Verification items for the finished model (mm, model axes). Face numbers are marked on the shaded views. A direction names the side the tool comes from. Give positions to 0.01 mm unless a question says otherwise; leave off trailing zeros. Write each loop counter-clockwise with the first axis right and the second up, starting at its lowest first coordinate (ties: lowest second). Pieces come first, ordered by that corner, then holes.
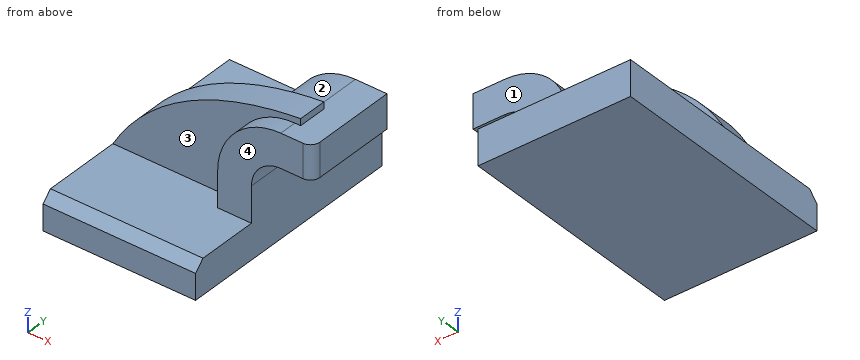
from build123d import *

# Parameters (mm, degrees)
F1_DEPTH = 63.5
F0_W     = 13.9366841115
F0_H     = 18.2897937342
F2_DEPTH = 25.4
F3_DEPTH = 15.875
F4_SIZE  = 5.08
F5_R     = 5.08


with BuildPart() as f1:
    # F0 (on Front) → F1 (new body, symmetric)
    with BuildSketch(Plane.XZ):
        Polygon((22.9852062658, 9.525), (-41.275, 9.525), (-41.275, -9.525), (41.275, -9.525), (41.275, 9.525), align=None)
    extrude(amount=F1_DEPTH, both=True)

    # F0 (on Front) → F2 (join, symmetric)
    with BuildSketch(Plane.XZ):
        with BuildLine():
            Line((22.9852062658, 28.8565382361), (22.9852062658, 9.525))
            Line((22.9852062658, 9.525), (41.275, 9.525))
            Line((41.275, 9.525), (41.275, 28.8565382361))
            ThreePointArc((41.275, 28.8565382361), (45.9246798487, 40.0818583875), (57.15, 44.7315382361))
            Line((57.15, 44.7315382361), (60.325, 44.7315382361))
            Line((60.325, 44.7315382361), (60.325, 63.0213319704))
            Line((60.325, 63.0213319704), (57.15, 63.0213319704))
            ThreePointArc((57.15, 63.0213319704), (32.9918426727, 53.0146955635), (22.9852062658, 28.8565382361))
        make_face()
        with Locations((67.2933420557, 53.8764351033)):
            Rectangle(F0_W, F0_H)
    extrude(amount=F2_DEPTH, both=True)

    # F0 (on Front) → F3 (join)
    with BuildSketch(Plane.XZ):
        with BuildLine():
            add(Edge.make_bspline(
                [(-41.275, 9.525), (-18.0427934974, 50.5091771483), (24.8379260302, 63.2460191846), (60.325, 66.675)],
                knots=[0, 0, 0, 0, 116.5705044169, 116.5705044169, 116.5705044169, 116.5705044169], degree=3))
            Line((-41.275, 9.525), (22.9852062658, 9.525))
            Line((22.9852062658, 9.525), (22.9852062658, 28.8565382361))
            ThreePointArc((22.9852062658, 28.8565382361), (32.9918426727, 53.0146955635), (57.15, 63.0213319704))
            Line((57.15, 63.0213319704), (60.325, 63.0213319704))
            Line((60.325, 63.0213319704), (60.325, 66.675))
        make_face()
    extrude(amount=F3_DEPTH)

    # F4
    f4_edges = [f1.edges().sort_by_distance(p)[0] for p in [
        (0, -63.5, 9.525),
    ]]
    chamfer(f4_edges, length=F4_SIZE)

    # F5
    f5_edges = [f1.edges().sort_by_distance(p)[0] for p in [
        (74.261684, -25.4, 53.876435),
    ]]
    fillet(f5_edges, radius=F5_R)


solid = f1.part
Item 1: Sectioned sample at C-C on y = 29. Record the cut outline in (x, z) (3 decimals).
Answer key:
outline: (-41.275, -9.525) - (41.275, -9.525) - (41.275, 9.525) - (-41.275, 9.525) - close
Item 2: Sectioned sample at B-B on z = 2. Record the cut outline in (x, y) (3 decimals).
Answer key:
outline: (-41.275, -63.5) - (41.275, -63.5) - (41.275, 63.5) - (-41.275, 63.5) - close
Item 3: Scan lines: line 1 along Z through (x, y) = (12, -27.5) (3 decimals); line 2 along Y through (x, z) = (36, 37.5); line 3 along Y through (x, z) = (14, 36) (3 decimals). Record each from-to range of solid material in increasing order.
Answer key:
line 1: z = -9.525 to 9.525
line 2: y = -25.4 to 25.4
line 3: y = -15.875 to 0
Item 4: Set-up check for the marked faces 1, 2, 3 and 4: record each of +Z, -Z, +X, -X, +Y, -Y from which the full face is reachable in a straight line by a thin tool's end or side.
Answer key:
face 1: +Z, +X, -X, +Y
face 2: +Z, -X, +Y
face 3: +Z, -X, -Y
face 4: +Z, +X, -X, -Y
Item 5: Sectioned sample at A-A on y = 8.5. Record the cut outline in (x, z) (3 decimals), then the cut area to 3 significant figures.
Answer key:
outline: (-41.275, -9.525) - (41.275, -9.525) - (41.275, 28.857) arc R15.875 cw to (57.15, 44.732) - (74.262, 44.732) - (74.262, 63.021) - (57.15, 63.021) arc R34.165 ccw to (22.985, 28.857) - (22.985, 9.525) - (-41.275, 9.525) - close
area: 2,960 mm2
Item 6: Depth check by flat-ended pin: pin 1 (21.5 mm diameter, centred on x = 7.5, y = -38, fed in from +Z) (3 decimals); pin 2 (8.5 mm diameter, centred on x = 69.5, y = -6.5, fed in from -Z); pin 3 (12 mm diameter, centred on x = -24, z = 40, fed in from +Y). Enter the tip coordinate at first touch or a pass-through.
Answer key:
pin 1: stops at z = 9.525
pin 2: stops at z = 44.73
pin 3: stops at y = 0
